For this review, take the finished solid that the model builds, in its own axes (mm). A direction names the side the tool comes from. Round coordinates to 2 decimals unless told otherwise and drop trailing zeros. Write each loop counter-clockwise with the first axis right and the second up, starting at its lowest first coordinate (ties: lowest second). Pieces come first, ordered by that corner, then holes. Notation, with made-up numbers: (-30.5, 78.5) - (17.5, 78.5) arc R36 ccw to (17.5, 116.5) - close; hole circle Ø5 at (-4, 65.5). An arc over 180 degrees is marked (long way). One line per item, written item: value. Start each with the question number.
Q1. Add section A-A on z = 1.35. Write out the cut boundary in (x, y).
Q2. Clearance check with flat-ended pins moving along their axes: pin 1 Ø0.6 at (x, z) = (23.5, 1) entering from +Y; pin 2 Ø2 at (x, z) = (3.5, 0.5) entering from +Y. State where each tip first meets the part, or that it passes through.
Q3. For probe 1 along X at (y, z) = (-8.5, 2.6); probe 2 along Y at (x, z) = (20, 3.9); probe 3 along Y at (x, z) = (23.25, 4.45), list the stretches that pass through material, from the lowest coordinate up.
Q4. Add section C-C on x = 24. Write out the cut boundary in (y, z).
Q5. Tool access review of faces 1 (the face through (25.48, -40.095, 0.986)), 2 (the face through (3.85, -19, 2)), 3 (the face through (13, -22, 0)): name each direction out of +Z, -Z, +X, -X, +Y, -Y from which nothing blocks a thin tool from reaching the whole face with its end or side.
Q6. Mouldability with a two-part tool opening along Y and no side actions: class faces 4 (the face through (13, -45, 2)), 5 (the face through (5.95, -5.85, 2.46)), 6 (the face through (0, -25, 2)) as +Y half, -Y half, draft (parallel to the pull), parting line (faces both ways), or undercut.
Q7. Add section B-B on y = -19.5. Write out the cut boundary in (x, z).
Q8. Add section D-D on x = 14.5. Write out the cut boundary in (y, z), and give its area (3 significant figures).
```python
from build123d import *

# Parameters (mm, degrees)
F0_W     = 27
F0_H     = 45
F0_R     = 1.8
F1_DEPTH = 5
F3_DEPTH = 27
F4_DEPTH = 2
F5_SIZE  = 5


with BuildPart() as f1:
    # F0 (on Top) → F1 (new body)
    with BuildSketch(Plane.XY):
        with Locations((13.5, -22.5)):
            Rectangle(F0_W, F0_H)
        Polygon((0.709103, -41.5), (2.354552, -38.65), (5.645448, -38.65), (7.290897, -41.5), (5.645448, -44.35), (2.354552, -44.35), align=None, mode=Mode.SUBTRACT)
        Polygon((19.709103, -41.5), (21.354552, -38.65), (24.645448, -38.65), (26.290897, -41.5), (24.645448, -44.35), (21.354552, -44.35), align=None, mode=Mode.SUBTRACT)
        with BuildLine():
            Line((3.85, -29), (3.85, -8))
            ThreePointArc((3.85, -8), (6, -5.85), (8.15, -8))
            Line((8.15, -8), (8.15, -29))
            ThreePointArc((8.15, -29), (6, -31.15), (3.85, -29))
        make_face(mode=Mode.SUBTRACT)
        with BuildLine():
            Line((18.85, -29), (18.85, -8))
            ThreePointArc((18.85, -8), (21, -5.85), (23.15, -8))
            Line((23.15, -8), (23.15, -29))
            ThreePointArc((23.15, -29), (21, -31.15), (18.85, -29))
        make_face(mode=Mode.SUBTRACT)
        Polygon((24.645448, -38.65), (21.354552, -38.65), (19.709103, -41.5), (21.354552, -44.35), (24.645448, -44.35), (26.290897, -41.5), align=None)
        with Locations((23, -41.5)):
            Circle(F0_R, mode=Mode.SUBTRACT)
        Polygon((5.645448, -38.65), (2.354552, -38.65), (0.709103, -41.5), (2.354552, -44.35), (5.645448, -44.35), (7.290897, -41.5), align=None)
        with Locations((4, -41.5)):
            Circle(F0_R, mode=Mode.SUBTRACT)
    extrude(amount=F1_DEPTH)

    # F2 (on face) → F3 (cut, through all)
    with BuildSketch(Plane.YZ.offset(27)):
        with BuildLine():
            Line((-34.5, 5), (-37.5, 5))
            ThreePointArc((-37.5, 5), (-36, 3.5), (-34.5, 5))
        make_face()
    extrude(amount=-F3_DEPTH, mode=Mode.SUBTRACT)

    # F0 (on Top) → F4 (cut)
    with BuildSketch(Plane.XY):
        with Locations((4, -41.5)):
            Circle(F0_R)
        with Locations((23, -41.5)):
            Circle(F0_R)
        Polygon((5.645448, -38.65), (2.354552, -38.65), (0.709103, -41.5), (2.354552, -44.35), (5.645448, -44.35), (7.290897, -41.5), align=None)
        with Locations((4, -41.5)):
            Circle(F0_R, mode=Mode.SUBTRACT)
        Polygon((24.645448, -38.65), (21.354552, -38.65), (19.709103, -41.5), (21.354552, -44.35), (24.645448, -44.35), (26.290897, -41.5), align=None)
        with Locations((23, -41.5)):
            Circle(F0_R, mode=Mode.SUBTRACT)
    extrude(amount=F4_DEPTH, mode=Mode.SUBTRACT)

    # F5
    f5_edges = [f1.edges().sort_by_distance(p)[0] for p in [
        (0, 0, 2.5),
        (27, 0, 2.5),
    ]]
    chamfer(f5_edges, length=F5_SIZE)


solid = f1.part
```
Result set:
1. outline: (0, -45) - (27, -45) - (27, -5) - (22, 0) - (5, 0) - (0, -5) - close; hole (0.71, -41.5) - (2.35, -44.35) - (5.65, -44.35) - (7.29, -41.5) - (5.65, -38.65) - (2.35, -38.65) - close; hole (3.85, -29) arc R2.15 ccw to (8.15, -29) - (8.15, -8) arc R2.15 ccw to (3.85, -8) - close; hole (18.85, -29) arc R2.15 ccw to (23.15, -29) - (23.15, -8) arc R2.15 ccw to (18.85, -8) - close; hole (19.71, -41.5) - (21.35, -44.35) - (24.65, -44.35) - (26.29, -41.5) - (24.65, -38.65) - (21.35, -38.65) - close
2. pin 1: stops at y = -1.2
2. pin 2: stops at y = -0.5
3. probe 1: x = 0 to 3.85, 8.15 to 18.85, 23.15 to 27
3. probe 2: y = -45 to -37.02, -34.98 to -30.9, -6.1 to 0
3. probe 3: y = -45 to -43.28, -39.72 to -37.4, -34.6 to -1.25
4. outline: (-45, 0) - (-44.35, 0) - (-44.35, 2) - (-43, 2) - (-43, 5) - (-45, 5) - close; (-40, 2) - (-38.65, 2) - (-38.65, 0) - (-2, 0) - (-2, 5) - (-34.5, 5) arc R1.5 cw to (-37.5, 5) - (-40, 5) - close
5. face 1: -Z
5. face 2: +Z, -Z
5. face 3: -Z, +X, -X, +Y, -Y
6. face 4: -Y half
6. face 5: undercut
6. face 6: draft
7. outline: (0, 0) - (3.85, 0) - (3.85, 5) - (0, 5) - close; (8.15, 0) - (18.85, 0) - (18.85, 5) - (8.15, 5) - close; (23.15, 0) - (27, 0) - (27, 5) - (23.15, 5) - close
8. outline: (-45, 0) - (0, 0) - (0, 5) - (-34.5, 5) arc R1.5 cw to (-37.5, 5) - (-45, 5) - close
8. area: 221 mm^2
